Input: part model. Units: mm. Frame: model coordinates. Face numbers are marked on the shaded views. A direction names the side the tool comes from. Round coordinates to 2 decimals unless told otherwise and drop trailing zeros. Order: outer loops, then holes, each group sorted by start corner. A loop starts at its lowest first (then second) coordinate and runs counter-clockwise, first axis right, second up.
Item 1: Mould query, pull axis X, two halves, no side actions, for the marked faces 3 and 4. Classes: released by +X, released by -X, zero draft, split by the parting line, or undercut.
Item 2: Cut plane A-A on z = 16. Output: boundary loops of the cut face in (x, y), then the cut area to 3 significant figures.
Item 3: Line query: L1, parallel to Y at x = 0, z = 50.25; L2, parallel to X at y = 0, z = 29; L3, parallel to X at y = 34.5, z = 3. Output: solid intervals per line, ascending.
Item 4: First-contact query: pin 1 (1.5 mm diameter, centred on y = -8, z = 27, fed in from +X); pin 2 (6 mm diameter, centred on y = 7.5, z = 17.5, fed in from -X); pin 3 (8 mm diameter, centred on y = 14, z = 26, fed in from -X). Flat tips, straight axial feed; report the tip coordinate or a pass-through.
Item 5: Reachability of the marked faces 1 and 2 from +Z, -Z, +X, -X, +Y, -Y: full face, straight path, thin tool, end or side. Return the list, or none.
Item 6: Cut plane B-B on z = 49.5. Output: boundary loops of the cut face in (x, y).
```python
from build123d import *

# Parameters (mm, degrees)
FILLET_R     = 3
CHAMFER_SIZE = 2


with BuildPart() as part:
    # Sketch → Revolution (revolve)
    with BuildSketch(Plane.XZ):
        Polygon((52, 0), (52, 35), (47.5, 41.426666), (47.5, 60), (50.5, 60), (50.5, 41.426666), (55, 35), (55, 0), align=None)
    revolve(axis=Axis((0, 0, 0), (0, 0, 1)))

    # Fillet
    fillet_edges = [part.edges().sort_by_distance(p)[0] for p in [
        (-50.5, 0, 41.426666),
        (-55, 0, 35),
        (52.75, 0, 38.213333),
        (-52, 0, 35),
        (-47.5, 0, 41.426666),
        (49.75, 0, 38.213333),
    ]]
    fillet(fillet_edges, radius=FILLET_R)

    # Chamfer
    chamfer_edges = [part.edges().sort_by_distance(p)[0] for p in [
        (-55, 0, 0),
    ]]
    chamfer(chamfer_edges, length=CHAMFER_SIZE)


solid = part.part
```
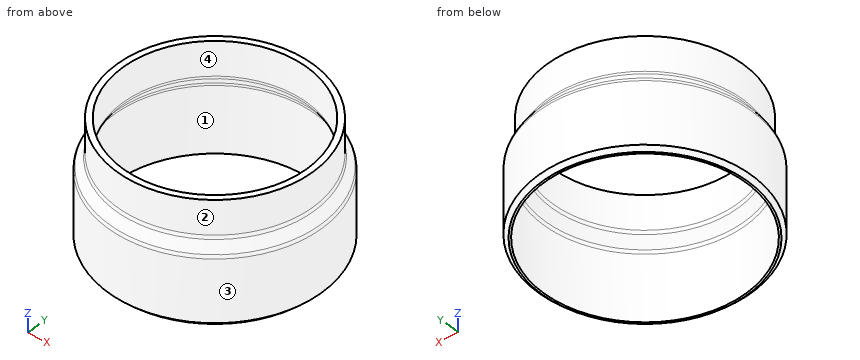
From the geometry:
1. face 3: split by the parting line
1. face 4: undercut
2. outline: circle Ø110 at (0, 0); hole circle Ø104 at (0, 0)
2. area: 1,010 mm2
3. L1: y = -50.5 to -47.5, 47.5 to 50.5
3. L2: x = -55 to -52, 52 to 55
3. L3: x = -42.83 to -38.91, 38.91 to 42.83
4. pin 1: stops at x = 54.52
4. pin 2: stops at x = -54.82
4. pin 3: stops at x = -54.08
5. face 1: -Z
5. face 2: +Z
6. outline: circle Ø101 at (0, 0); hole circle Ø95 at (0, 0)
